Autodesk Inventor part; units mm, degrees
ref_plane "YZ Plane" through (0, 0, 0) normal (1, 0, 0) x (0, 1, 0)
ref_plane "XZ Plane" through (0, 0, 0) normal (0, 1, 0) x (-1, 0, 0)
ref_plane "XY Plane" through (0, 0, 0) normal (0, 0, 1) x (1, 0, 0)
sketch "Sketch1" plane through (0, 0, 0) normal (0, 0, 1) x (1, 0, 0)
  line L0 (0, 15.875) -> (3.175, 15.875)
  line L1 (3.175, 15.875) -> (3.175, 19.05)
  line L2 (3.175, 19.05) -> (6.35, 15.875)
  line L3 (6.35, 15.875) -> (6.35, 9.525)
  line L4 (6.35, 9.525) -> (3.175, 6.35)
  line L5 (3.175, 6.35) -> (3.175, 9.525)
  line L6 (3.175, 9.525) -> (0, 9.525)
  line L7 (9.525, 0) -> (9.525, 3.175)
  line L8 (9.525, 3.175) -> (6.35, 3.175)
  line L9 (6.35, 3.175) -> (9.525, 6.35)
  line L10 (9.525, 6.35) -> (15.875, 6.35)
  line L11 (15.875, 6.35) -> (19.05, 3.175)
  line L12 (19.05, 3.175) -> (15.875, 3.175)
  line L13 (15.875, 3.175) -> (15.875, 0)
  line L14 (25.4, 9.525) -> (22.225, 9.525)
  line L15 (22.225, 9.525) -> (22.225, 6.35)
  line L16 (22.225, 6.35) -> (19.05, 9.525)
  line L17 (19.05, 9.525) -> (19.05, 15.875)
  line L18 (19.05, 15.875) -> (22.225, 19.05)
  line L19 (22.225, 19.05) -> (22.225, 15.875)
  line L20 (22.225, 15.875) -> (25.4, 15.875)
  line L21 (15.875, 25.4) -> (15.875, 22.225)
  line L22 (15.875, 22.225) -> (19.05, 22.225)
  line L23 (19.05, 22.225) -> (15.875, 19.05)
  line L24 (15.875, 19.05) -> (9.525, 19.05)
  line L25 (9.525, 19.05) -> (6.35, 22.225)
  line L26 (6.35, 22.225) -> (9.525, 22.225)
  line L27 (9.525, 22.225) -> (9.525, 25.4)
  circle A0 centre (12.7, 12.7) radius 3.175
  line L28 (0, 23.8125) -> (0, 15.875)
  line L29 (0, 9.525) -> (0, 1.5875)
  line L30 (9.525, 0) -> (1.5875, 0)
  line L31 (15.875, 0) -> (23.8125, 0)
  line L32 (25.4, 1.5875) -> (25.4, 9.525)
  line L33 (25.4, 15.875) -> (25.4, 23.8125)
  line L34 (23.8125, 25.4) -> (15.875, 25.4)
  line L35 (9.525, 25.4) -> (1.5875, 25.4)
  arc A1 (0, 1.5875) -> (1.5875, 0) centre (1.5875, 1.5875) ccw
  arc A2 (1.5875, 25.4) -> (0, 23.8125) centre (1.5875, 23.8125) ccw
  arc A3 (25.4, 23.8125) -> (23.8125, 25.4) centre (23.8125, 23.8125) ccw
  arc A4 (23.8125, 0) -> (25.4, 1.5875) centre (23.8125, 1.5875) ccw
  point P0 (0, 0)
  point P1 (25.4, 0)
  point P2 (0, 25.4)
  dimension "d5" = 6.35
  dimension "d7" = 12.7
  dimension "d8" = 3.175
  dimension "d9" = 3.175
  dimension "d13" = 360
  dimension "d15" = 6.35
  dimension "d16" = 1.5875
extrude "Extrusion2" add sketch "Sketch1" against normal blind 88.9
properties part number "5 in shooter standoff"
Could you check a few things on this model? Use its own coordinates, in mm. A direction names the side the tool comes from. Round coordinates to 2 decimals unless told otherwise and drop trailing zeros. Loops run counter-clockwise (first coordinate to the right, second up) from the corner with the lowest first, then second, coordinate; pieces in that order, holes last.
Q1. Thinking about a two-plate mould opening in X: for faces 1 (the flat face through (8, 22.225, -44)), 2 (the flat face through (24, 9.525, -44)), 3 (the flat face through (25.4, 6, -44)), which applies, pulls with the +X half, pulls with the -X half, needs draft (parallel to the pull), parting line crosses it, or undercut?
Q2. I want a section at D-D (x = 17.25). Write out the boundary of the cut face in (y, z) (3 decimals).
Q3. On a 3-axis mill with a long thin cutter (end or side, diameter ignored), from which of +Z, -Z, +X, -X, +Y, -Y can I reach the whole of each face in a straight line? I mean faces 4 (the flat face through (15.875, 24, -44)), 5 (the flat face through (24, 15.875, -44)), 6 (the flat face through (9.525, 2, -44)). Say none if no direction works.
Q4. For P1, Ø1.9, axis at y = 13.5, z = -25.5, coming from the -X side; P2, Ø5, axis at x = 12.5, z = -23.5, coming from the +Y side, each with a flat end and sliding along its axis, tell me the tip position at first contact or that it passes through.
Q5. I want a section at A-A (x = 12.7). Write out the boundary of the cut face in (y, z) (3 decimals), and give its area (3 significant figures).
Q6. I want a section at C-C (y = 18). Write out the boundary of the cut face in (x, z) (3 decimals).
Q7. Please list where these lines run through material, in increasing order: L1, parallel to X at y = 23.5, z = -54.5 (3 decimals); L2, parallel to X at y = 17.5, z = -42 (3 decimals).
Answer below:
1. face 1: undercut
1. face 2: needs draft
1. face 3: pulls with the +X half
2. outline: (0, -88.9) - (3.175, -88.9) - (3.175, 0) - (0, 0) - close; (4.975, -88.9) - (20.425, -88.9) - (20.425, 0) - (4.975, 0) - close; (22.225, -88.9) - (25.4, -88.9) - (25.4, 0) - (22.225, 0) - close
3. face 4: +Z, -Z, +Y
3. face 5: +Z, -Z, +X
3. face 6: +Z, -Z, -Y
4. P1: stops at x = 6.35
4. P2: stops at y = 19.05
5. outline: (6.35, -88.9) - (9.525, -88.9) - (9.525, 0) - (6.35, 0) - close; (15.875, -88.9) - (19.05, -88.9) - (19.05, 0) - (15.875, 0) - close
5. area: 565 mm2
6. outline: (0, -88.9) - (3.175, -88.9) - (3.175, 0) - (0, 0) - close; (4.225, -88.9) - (21.175, -88.9) - (21.175, 0) - (4.225, 0) - close; (22.225, -88.9) - (25.4, -88.9) - (25.4, 0) - (22.225, 0) - close
7. L1: x = 0 to 9.525, 15.875 to 25.4
7. L2: x = 0 to 3.175, 4.725 to 20.675, 22.225 to 25.4
